Source: CAD feature listing. Evaluate the final solid. Frame: model axes, mm. A direction names the side the tool comes from. Coordinates: 2 decimals unless noted, no trailing zeros. Loops run counter-clockwise (first coordinate to the right, second up) from the corner with the lowest first, then second, coordinate; pieces in that order, holes last.
Item 1: Line query: probe 1 along Z at (x, y) = (1.5, 12.75); probe 2 along Z at (x, y) = (-3.25, 16.75); probe 3 along Y at (x, z) = (3.1, 0). Output: solid intervals per line, ascending.
Item 2: Reachability of faces 5 (the flat face through (-8, 12, -7)), 6 (the flat face through (0, 11.25, 11)), 7 (the flat face through (2.5, 11, -1)) from +Z, -Z, +X, -X, +Y, -Y: full face, straight path, thin tool, end or side. Return the list, or none.
Item 3: Section query C-C, the plane y = 12.5. State how many separate pieces and enclosed holes the cut face has, then the cut area to 4 significant figures.
Item 4: Section query A-A, the plane x = -5. Return the cut outline in (y, z), then the cut area to 3 significant figures.
Item 5: Pin query (flat end, axial travel): pin 1 Ø1.2 at (x, z) = (0, -11) entering from -Y; pin 2 Ø5 at (x, z) = (-1.5, -3.5) entering from +Y; pin 3 Ø3 at (y, z) = (11.5, 1) entering from -X; pin 4 Ø6 at (x, y) = (-11, 12.5) entering from -Z. Return the tip coordinate at first contact, or that it passes through.
Item 6: Pull-direction query (Y, two-part tool) for faces 1 (the flat face through (2, 0, 0)), 2 (the flat face through (-5, 12, 10)), 3 (the cylindrical face through (-10.46, 10.06, 8.48)), 4 (the flat face through (1.2, 15.1, -1.5)); classes: +Y half, -Y half, draft (parallel to the pull), parting line (faces both ways), or undercut.
Item 7: Section query B-B, the plane x = -11. Return the cut outline in (y, z).
Item 8: Section query D-D, the plane z = 8. Return the cut outline in (x, y).
```python
from build123d import *

# Parameters (mm, degrees)
EXTRUDE_1_DEPTH     = 25
CUT_EXTRUDE_1_DEPTH = 2.5
SKETCH_3_R          = 1.6
CUT_EXTRUDE_2_DEPTH = 2.5
EXTRUDE_2_DEPTH     = 2.5
SKETCH_5_R          = 2.5
CUT_EXTRUDE_3_DEPTH = 37.827299657


with BuildPart() as part:
    # Эскиз1 → Бобышка-Вытянуть1 (new body)
    with BuildSketch(Plane(origin=(0, 0, 0), x_dir=(1, 0, 0), z_dir=(0, 1, 0))):
        Polygon((0, 7), (0, -7), (-15, -7), (-15, -10), (5, -10), (5, 10), (-15, 10), (-15, 7), align=None)
    extrude(amount=EXTRUDE_1_DEPTH)

    # Эскиз2 → Вырез-Вытянуть1 (cut)
    with BuildSketch(Plane.ZY):
        Polygon((3, 14.232050808), (0, 15.964101615), (-3, 14.232050808), (-3, 10.767949192), (0, 9.035898385), (3, 10.767949192), align=None)
    extrude(amount=-CUT_EXTRUDE_1_DEPTH, mode=Mode.SUBTRACT)

    # Эскиз3 → Вырез-Вытянуть2 (cut)
    with BuildSketch(Plane.ZY.offset(-2.5)):
        with Locations((0, 12.5)):
            Circle(SKETCH_3_R)
    extrude(amount=-CUT_EXTRUDE_2_DEPTH, mode=Mode.SUBTRACT)

    # Эскиз4 → Бобышка-Вытянуть2 (add)
    with BuildSketch(Plane(origin=(0, 0, -10), x_dir=(-1, 0, 0), z_dir=(0, 0, -1))):
        with BuildLine():
            Line((-2.5, 13.75), (2.5, 13.75))
            ThreePointArc((2.5, 13.75), (3.75, 12.5), (2.5, 11.25))
            Line((2.5, 11.25), (-2.5, 11.25))
            ThreePointArc((-2.5, 11.25), (-3.75, 12.5), (-2.5, 13.75))
        make_face()
    extrude_2 = extrude(amount=EXTRUDE_2_DEPTH)

    # Зеркальное отражение1: Бобышка-Вытянуть2 across plane
    add(extrude_2.mirror(Plane(origin=(0, 0, 0), x_dir=(1, 0, 0), z_dir=(0, 0, -1))))

    # Эскиз5 → Вырез-Вытянуть3 (cut, through all)
    with BuildSketch(Plane(origin=(0, 0, -10), x_dir=(-1, 0, 0), z_dir=(0, 0, -1))):
        with Locations((11, 12.5)):
            Circle(SKETCH_5_R)
    extrude(amount=-CUT_EXTRUDE_3_DEPTH, mode=Mode.SUBTRACT)


solid = part.part
```
Verdict:
1. probe 1: z = -12.5 to -3, 3 to 12.5
1. probe 2: z = -10 to -7, 7 to 10
1. probe 3: y = 0 to 10.9, 14.1 to 25
2. face 5: -X, +Y, -Y
2. face 6: +Z, +X, -X, -Y
2. face 7: -X
3. separate pieces: 4
3. enclosed holes: 0
3. area: 174.5 mm2
4. outline: (0, -10) - (25, -10) - (25, -7) - (0, -7) - close; (0, 7) - (25, 7) - (25, 10) - (0, 10) - close
4. area: 150 mm2
5. pin 1: stops at y = 11.25
5. pin 2: stops at y = 25
5. pin 3: stops at x = 2.5
5. pin 4: stops at z = -10
6. face 1: -Y half
6. face 2: draft
6. face 3: undercut
6. face 4: undercut
7. outline: (0, -10) - (10, -10) - (10, -7) - (0, -7) - close; (0, 7) - (10, 7) - (10, 10) - (0, 10) - close; (15, -10) - (25, -10) - (25, -7) - (15, -7) - close; (15, 7) - (25, 7) - (25, 10) - (15, 10) - close
8. outline: (-15, 0) - (5, 0) - (5, 25) - (-15, 25) - close; hole circle Ø5 at (-11, 12.5)
